from build123d import *

# Parameters (mm, degrees)
SKETCH_1_R      = 1.5
EXTRUDE_1_DEPTH = 13
EXTRUDE_2_DEPTH = 12
FILLET_1_R      = 0.5


with BuildPart() as part:
    # 草图1 → 凸台-拉伸1 (new body)
    with BuildSketch(Plane.XY):
        Circle(SKETCH_1_R)
    extrude(amount=EXTRUDE_1_DEPTH)

    # 草图2 → 凸台-拉伸2 (add)
    with BuildSketch(Plane.XY):
        Polygon((0, 1.5), (8.1, 1.5), (8.1, 0.83), (8.77, 0.83), (8.77, 0.16), (9.44, 0.16), (9.44, -0.51), (10.11, -0.51), (10.11, -2.5), (0, 0), align=None)
    extrude(amount=EXTRUDE_2_DEPTH)

    # 圆角1
    fillet_1_edges = [part.edges().sort_by_distance(p)[0] for p in [
        (10.11, -2.5, 6),
    ]]
    fillet(fillet_1_edges, radius=FILLET_1_R)


solid = part.part
For this review, take the finished solid that the model builds, in its own axes (mm). A direction names the side the tool comes from. Coordinates: 2 decimals unless noted, no trailing zeros. Loops run counter-clockwise (first coordinate to the right, second up) from the corner with the lowest first, then second, coordinate; pieces in that order, holes last. Notation, with made-up numbers: (-22.75, -9) -> (-4.75, -9) arc R4 ccw to (-4.75, -2) -> close; hole circle Ø10 at (-1, 5). An arc over 180 degrees is marked (long way). Write each question's results on one line, items separated by ' | '.
Q1. Machinability: for faces 1 (the flat face through (5.529, -1.367, 5.916)), 2 (the flat face through (10.11, -1, 6)), which of the approach directions +Z, -Z, +X, -X, +Y, -Y give a long, thin tool a straight path to every point of the face, cutting with its end or side? Answer none if there is none.
Taken from the geometry:
face 1: +Z, -Z, -Y | face 2: +Z, -Z, +X, +Y, -Y
Q2. Add section C-C, the plane x = 0.5. State the section outline as (y, z) points.
Taken from the geometry:
outline: (-1.41, 0) -> (1.5, 0) -> (1.5, 12) -> (1.41, 12) -> (1.41, 13) -> (-1.41, 13) -> close
Q3. Add section A-A, the plane y = -0.7. State the section outline as (x, z) points, then the cut area to 3 significant figures.
Taken from the geometry:
outline: (-1.33, 0) -> (1.33, 0) -> (1.33, 13) -> (-1.33, 13) -> close; (2.83, 0) -> (10.11, 0) -> (10.11, 12) -> (2.83, 12) -> close | area: 122 mm²
Q4. Add section B-B, the plane z = 6.5. State the section outline as (x, y) points.
Taken from the geometry:
outline: (0, 1.5) arc R1.5 ccw (long way) to (1.46, -0.36) -> (9.49, -2.35) arc R0.5 ccw to (10.11, -1.86) -> (10.11, -0.51) -> (9.44, -0.51) -> (9.44, 0.16) -> (8.77, 0.16) -> (8.77, 0.83) -> (8.1, 0.83) -> (8.1, 1.5) -> close
Q5. For pin 1 Ø3 at (x, z) = (6, 2) entering from -Y; pin 2 Ø6 at (x, z) = (1.5, 7.5) entering from -Y, all flat-tipped, find the tip position at first contact; note any pin that passes through.
Taken from the geometry:
pin 1: y = -1.85 | pin 2: y = -1.5
Q6. Add section D-D, the plane y = 0. State the section outline as (x, z) points.
Taken from the geometry:
outline: (-1.5, 0) -> (9.44, 0) -> (9.44, 12) -> (1.5, 12) -> (1.5, 13) -> (-1.5, 13) -> close
Q7. To check wall thickness, follow line 1 along X through (y, z) = (0, 7.75); line 2 along Z through (x, y) = (9.75, -1.3); line 3 along Y through (x, z) = (6.25, 10). State the ranges of each line that lie inside material, in increasing order. Write a range as [from, to].
Taken from the geometry:
line 1: [-1.5, 9.44] | line 2: [0, 12] | line 3: [-1.55, 1.5]
